Autodesk Inventor part; units mm, degrees
ref_plane "YZ Plane" through (0, 0, 0) normal (1, 0, 0) x (0, 1, 0)
ref_plane "XZ Plane" through (0, 0, 0) normal (0, 1, 0) x (-1, 0, 0)
ref_plane "XY Plane" through (0, 0, 0) normal (0, 0, 1) x (1, 0, 0)
sketch "Sketch2" plane through (0, 0, 0) normal (0, 1, 0) x (-1, 0, 0)
  line L0 (0, 0) -> (6.25, 0)
  line L1 (6.25, 0) -> (6.25, -240)
  line L2 (6.25, -240) -> (0, -240)
  line L3 (0, -240) -> (0, 0)
  line L4 (0, 0) -> (11.25, 0)
  line L5 (11.25, 0) -> (11.25, 5)
  line L6 (11.25, 5) -> (0, 5)
  line L7 (0, 5) -> (0, 0)
  line L8 (0, -240) -> (11.25, -240)
  line L9 (11.25, -240) -> (11.25, -245)
  line L10 (11.25, -245) -> (0, -245)
  line L11 (0, -245) -> (0, -240)
  dimension "d15" = 6.25
  dimension "d16" = 240
  dimension "d17" = 11.25
  dimension "d18" = 5
  dimension "d19" = 5
revolve "Revolution1" add sketch "Sketch2" angle 360 about axis through (0, 0, -240) along (0, 0, 1)
sketch "Sketch3" plane through (0, 0, 5) normal (0, 0, 1) x (1, 0, 0)
  line L0 (-10, -0.0006) -> (-5.0005, 8.66)
  line L1 (-5.0005, 8.66) -> (4.9995, 8.6606)
  line L2 (4.9995, 8.6606) -> (10, 0.0006)
  line L3 (10, 0.0006) -> (5.0005, -8.66)
  line L4 (5.0005, -8.66) -> (-4.9995, -8.6606)
  line L5 (-4.9995, -8.6606) -> (-10, -0.0006)
  point P0 (0, 0)
  point P1 (0, 0)
  dimension "d21" = 10
extrude "Extrusion1" add sketch "Sketch3" along normal blind 15
sketch "Sketch4" plane through (0, 0, -245) normal (0, 0, -1) x (-1, 0, 0)
  line L0 (-5, -8.6603) -> (-10, 0)
  line L1 (-10, 0) -> (-5, 8.6603)
  line L2 (-5, 8.6603) -> (5, 8.6603)
  line L3 (5, 8.6603) -> (10, 0)
  line L4 (10, 0) -> (5, -8.6603)
  line L5 (5, -8.6603) -> (-5, -8.6603)
  point P0 (0, 0)
  point P1 (0, 0)
  dimension "d24" = 10
extrude "Extrusion2" add sketch "Sketch4" along normal blind 15
fillet "Fillet1" radius 7 12 edges at (0, 8.6603, -260) (7.5, 4.3301, -260) (7.5, -4.3301, -260) (0, -8.6603, -260) (-7.5, -4.3301, -260) (-7.5, 4.3301, -260) (-7.5003, 4.3297, 20) (-0.0005, 8.6603, 20) (7.4997, 4.3306, 20) (7.5003, -4.3297, 20) (0.0005, -8.6603, 20) (-7.4997, -4.3306, 20)
sketch "Sketch5" plane through (0, 0, 20) normal (0, 0, 1) x (1, 0, 0)
  circle A0 centre (0, 0) radius 6.25
  circle A1 centre (0, 0) radius 1.5
  point P0 (0, 0)
  dimension "d28" = 3
extrude "Extrusion3" add sketch "Sketch5" along normal blind 10 contours A1
sketch "Sketch6" plane through (0, 0, -260) normal (0, 0, -1) x (-1, 0, 0)
  circle A0 centre (0, 0) radius 1.5
  dimension "d31" = 3
extrude "Extrusion4" add sketch "Sketch6" along normal blind 10
properties part number "Resistencia"
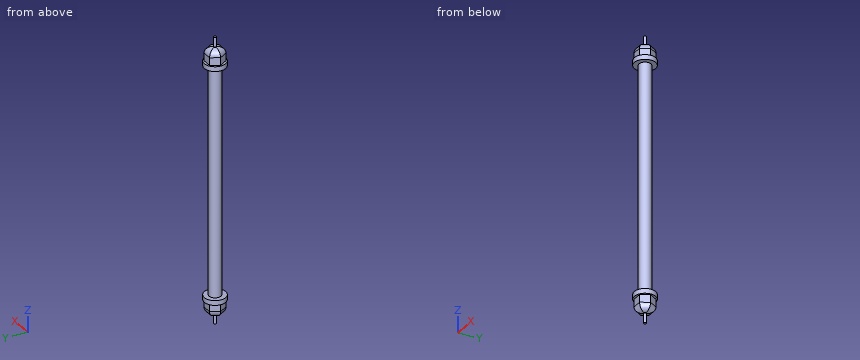
Geometry: final body of the model. Coordinates: model frame, mm. Round coordinates to 2 decimals unless told otherwise and drop trailing zeros. Order: outer loops, then holes, each group sorted by start corner. A loop starts at its lowest first (then second) coordinate and runs counter-clockwise, first axis right, second up. Notation, with made-up numbers: (60, 76) -> (92, 76) arc R29 ccw to (92, 103) -> close; hole circle Ø5 at (55, 85.25). An arc over 180 degrees is marked (long way). Use one line per item in the form item = value.
(1) Ray query, probe 1 along Z at (x, y) = (1, 9.75); probe 2 along Y at (x, z) = (-0.75, -183.5); probe 3 along Z at (x, y) = (-6.25, -2). Return the intervals inside material, ascending. Write a range as [from, to].
Results list:
probe_1 = [-245, -240], [0, 5]
probe_2 = [-6.2, 6.2]
probe_3 = [-258.14, -240], [0, 18.14]
(2) First-contact query: pin 1 Ø6 at (x, z) = (-6.5, -186) entering from +Y; pin 2 Ø3 at (x, y) = (8.5, 8.5) entering from -Z; pin 3 Ø1 at (x, y) = (-1.5, 6.5) entering from +Z; pin 4 Ø11 at (x, y) = (-3.5, -3) entering from +Z. Flat tips, straight axial feed; report the tip coordinate or a pass-through.
Results list:
pin_1 = 5.18
pin_2 = -245
pin_3 = 18.49
pin_4 = 30
(3) Section A-A on z = -76.5. Return loops of the section in (x, y).
Results list:
outline = circle Ø12.5 at (0, 0)
